from build123d import *

# Parameters (mm, degrees)
SKETCH1_W           = 3
SKETCH1_H           = 80
BOSS_EXTRUDE1_DEPTH = 3


with BuildPart() as part:
    # Sketch1 → Boss-Extrude1 (new body)
    with BuildSketch(Plane(origin=(0, 0, 0), x_dir=(1, 0, 0), z_dir=(0, 1, 0))):
        Polygon((-18, -40), (-18, -92), (18, -92), (18, -40), (15, -40), (15, 40), (18, 40), (18, 92), (-18, 92), (-18, 40), (-15, 40), (-15, -40), align=None)
        with Locations((16.5, 0)):
            Rectangle(SKETCH1_W, SKETCH1_H)
        with Locations((19.5, 0)):
            Rectangle(SKETCH1_W, SKETCH1_H)
        with Locations((-19.5, 0)):
            Rectangle(SKETCH1_W, SKETCH1_H)
        with Locations((-16.5, 0)):
            Rectangle(SKETCH1_W, SKETCH1_H)
    extrude(amount=BOSS_EXTRUDE1_DEPTH)


solid = part.part
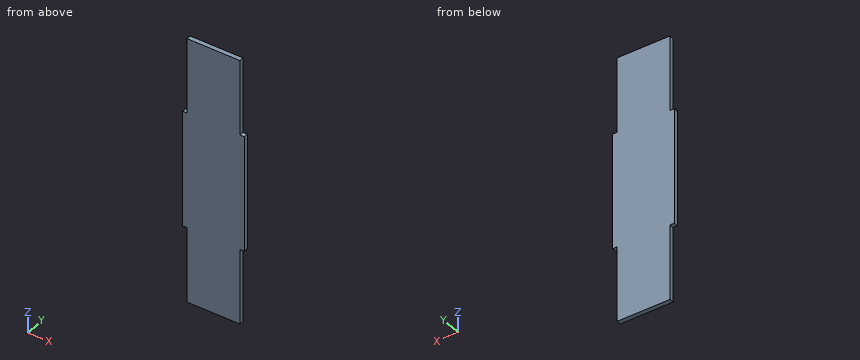
The listing builds one solid part. Answer for the finished solid, in the listing's coordinates (mm). Give positions to 0.01 mm unless a question says otherwise; leave off trailing zeros. Loops run counter-clockwise (first coordinate to the right, second up) from the corner with the lowest first, then second, coordinate; pieces in that order, holes last. Notation, with made-up numbers: (64.25, -6.75) - (69.25, -6.75) arc R13 ccw to (69.25, 15.25) - close; hole circle Ø5 at (55, 78). An arc over 180 degrees is marked (long way). Write each question's results on one line, items separated by ' | '.
1. Flat-ended cylindrical pins translate along their axes: P1, Ø1.5, axis at y = 2, z = 65.5, coming from the +X side; P2, Ø1.5, axis at x = -19.5, y = 1.5, coming from the +Z side; P3, Ø0.9, axis at x = 19.5, y = 1.5, coming from the -Z side. Find the tip coordinate at first contact, or state that the pin passes through.
Resolved:
P1: stops at x = 18 | P2: stops at z = 40 | P3: stops at z = -40
2. Consider probe 1 along X at (y, z) = (1.5, 44). Determine where the line is inside the solid, lowest interval first. Write a range as from..to.
Resolved:
probe 1: x = -18..18
3. Find section B-B, the plane z = -43.5. Write down the section's boundary in (x, y), then the cut area to 3 significant figures.
Resolved:
outline: (-18, 0) - (18, 0) - (18, 3) - (-18, 3) - close | area: 108 mm^2
4. Find section A-A, the plane y = 2.55. Write down the section's boundary in (x, z), then the cut area to 3 significant figures.
Resolved:
outline: (-21, -40) - (-18, -40) - (-18, -92) - (18, -92) - (18, -40) - (21, -40) - (21, 40) - (18, 40) - (18, 92) - (-18, 92) - (-18, 40) - (-21, 40) - close | area: 7,100 mm^2
